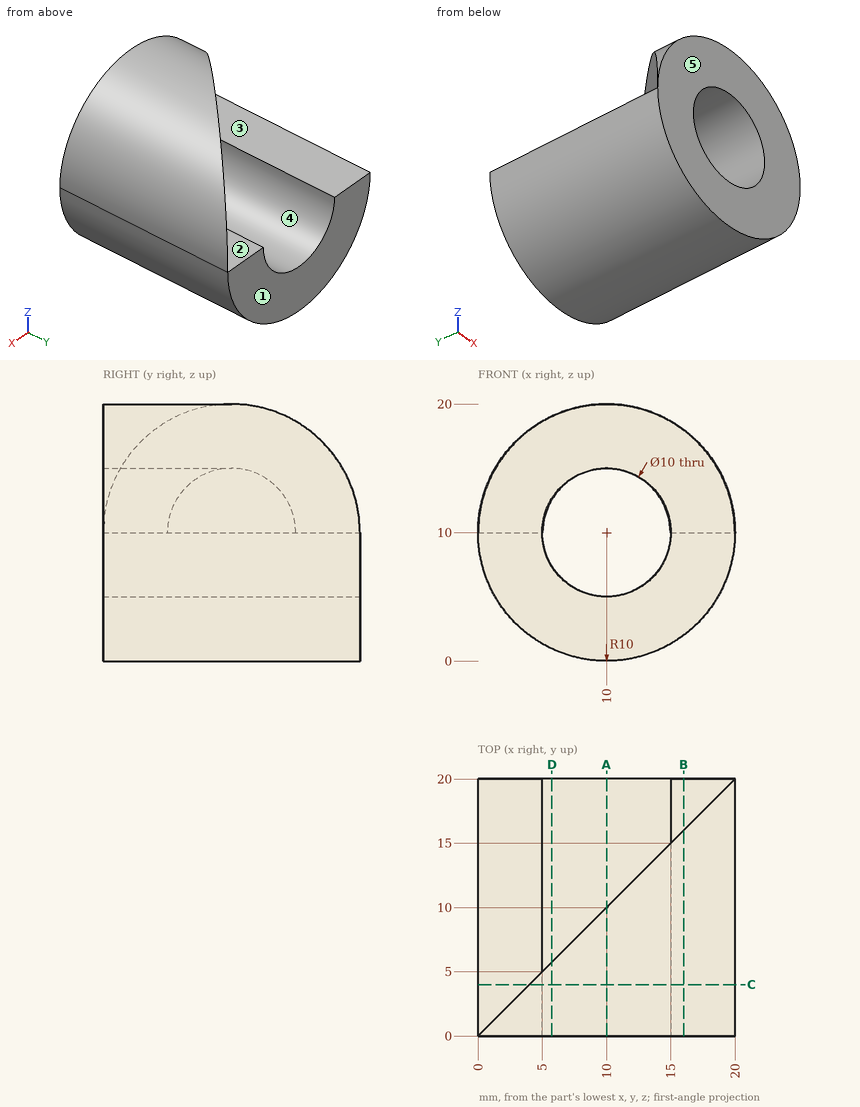
Source: three-view drawing plus pictorial views. Frame: mm from the lowest corner of the part. A direction names the side the tool comes from. Give positions to 0.01 mm unless a question says otherwise; leave off trailing zeros. Write each loop counter-clockwise with the first axis right and the second up, starting at its lowest first coordinate (ties: lowest second). Pieces come first, ordered by that corner, then holes. Notation, with made-up numbers: (22.25, -1.5) - (48.25, -1.5) arc R17 cw to (48.25, 8.5) - close; hole circle Ø1 at (50, 79). An arc over 180 degrees is marked (long way). Write item = value, one per line. Start each with the question number.
Q1. Reachability of the marked faces 1 and 2 from +Z, -Z, +X, -X, +Y, -Y: full face, straight path, thin tool, end or side. Return the list, or none.
Q2. Draft query along Z for the marked faces 3, 4 and 5. Return one class per face: +Z half, -Z half, draft (parallel to the pull), parting line (faces both ways), or undercut.
Q3. Cut plane B-B, the plane x = 16. Return loops of the section in (y, z).
Q4. Material intervals for probe 1 along Z at (x, y) = (10, 5.75); probe 2 along X at (y, z) = (6.75, 8); probe 3 along Z at (x, y) = (11, 10.5), sorted ascending.
Q5. Cut plane C-C, the plane y = 4. Return loops of the section in (x, z).
Q6. Cut plane D-D, the plane x = 5.75. Return loops of the section in (y, z), then the cut area to 3 significant figures.
Q7. Cut plane A-A, the plane x = 10. Return loops of the section in (y, z), then the cut area to 3 significant figures.
Q8. Pin query (flat end, axial travel): pin 1 Ø3 at (y, z) = (8, 16.5) entering from +X; pin 2 Ø3 at (x, z) = (10, 15) entering from +Y; pin 3 Ø1.5 at (x, y) = (18.5, 18) entering from +Z. Return the tip coordinate at first contact, or that it passes through.
Computed values:
q1.face_1 = +Z, -Z, +X, -X, +Y
q1.face_2 = +Z, -X, +Y
q2.face_3 = +Z half
q2.face_4 = undercut
q2.face_5 = draft
q3.outline = (0, 2) - (20, 2) - (20, 10) - (16, 10) - (16, 18) - (0, 18) - close
q4.probe_1 = 0 to 5, 15 to 20
q4.probe_2 = 0.2 to 5.42, 14.58 to 19.8
q4.probe_3 = 0.05 to 5.1, 14.9 to 19.95
q5.outline = (0, 10) arc R10 ccw (long way) to (4, 18) - (4, 10) - close; hole circle Ø10 at (10, 10)
q6.outline = (0, 0.95) - (20, 0.95) - (20, 7.37) - (0, 7.37) - close; (0, 12.63) - (5.75, 12.63) - (5.75, 19.05) - (0, 19.05) - close
q6.area = 165 mm²
q7.outline = (0, 0) - (20, 0) - (20, 5) - (0, 5) - close; (0, 15) - (10, 15) - (10, 20) - (0, 20) - close
q7.area = 150 mm²
q8.pin_1 = 18.66
q8.pin_2 = 11.5
q8.pin_3 = 16.28
